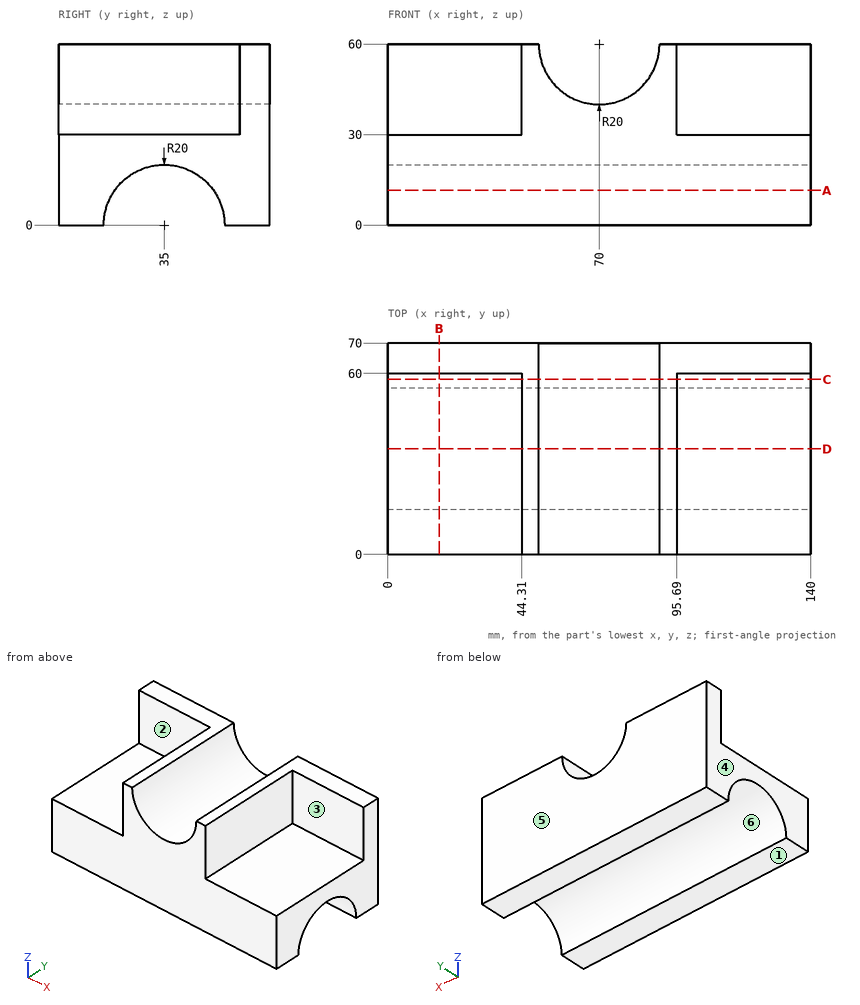
Part print with two shaded views. Sizes in mm from the minimum x, y, z corner. A direction names the side the tool comes from. Coordinates: 2 decimals unless noted, no trailing zeros. Order: outer loops, then holes, each group sorted by start corner. A loop starts at its lowest first (then second) coordinate and runs counter-clockwise, first axis right, second up. Notation, with made-up numbers: (-13, 69) - (9, 69) arc R19 ccw to (9, 90) - close; hole circle Ø4 at (-4, 27.5). An arc over 180 degrees is marked (long way). Write item = value, one per line. Start each with the question number.
1) Two-plate mould, pull along Y, no slides. Class the marked faces 4, 5 and 6: pulls with the +Y half, pulls with the -Y half, needs draft (parallel to the pull), parting line crosses it, or undercut.
2) Saw through at D-D on y = 35. Write the cut outline in (x, z).
3) Saw through at B-B on x = 17. Write the cut outline in (y, z), then the cut area to 3 significant figures.
4) Flat gauge pins, fed straight in: pin 1 Ø1 at (x, z) = (77.5, 9.5) entering from -Y; pin 2 Ø3 at (x, z) = (28.5, 50.5) entering from -Y; pin 3 Ø13.5 at (x, y) = (19.5, 22.5) entering from +Z; pin 4 Ø8 at (y, z) = (43.5, 37) entering from +X. Where does each tip first touch, or does it go through?
5) Saw through at A-A on z = 11.5. Write the cut outline in (x, y), then the cut area to 3 significant figures.
6) 3-axis set-ups, long thin cutter, end or side, ignore diameter. For the marked faces 1, 2 and 3: which of +Z, -Z, +X, -X, +Y, -Y reach the whole face in a straight line?
7) Wall check: line 1 along Y through (x, z) = (79, 4); line 2 along X through (y, z) = (11.5, 52.5); line 3 along X through (y, z) = (45.5, 43) (1 decimal). Give the ranges that are in metal, low to high. Write a range as from..to.
8) Saw through at C-C on y = 58. Write the cut outline in (x, z), then the cut area to 3 significant figures.
From the geometry:
q1.face_4 = needs draft
q1.face_5 = pulls with the +Y half
q1.face_6 = undercut
q2.outline = (0, 20) - (140, 20) - (140, 30) - (95.69, 30) - (95.69, 60) - (90, 60) arc R20 cw to (50, 60) - (44.31, 60) - (44.31, 30) - (0, 30) - close
q3.outline = (0, 0) - (15, 0) arc R20 cw to (55, 0) - (70, 0) - (70, 60) - (60, 60) - (60, 30) - (0, 30) - close
q3.area = 1,770 mm^2
q4.pin_1 = 0
q4.pin_2 = 60
q4.pin_3 = 30
q4.pin_4 = 95.69
q5.outline = (0, 0) - (140, 0) - (140, 18.64) - (0, 18.64) - close; (0, 51.36) - (140, 51.36) - (140, 70) - (0, 70) - close
q5.area = 5,220 mm^2
q6.face_1 = -Z, +X, -X, +Y, -Y
q6.face_2 = +Z, -X, -Y
q6.face_3 = +Z, +X, -Y
q7.line_1 = 0..15.4, 54.6..70
q7.line_2 = 44.31..51.46, 88.54..95.69
q7.line_3 = 44.3..59.5, 80.5..95.7
q8.outline = (0, 0) - (140, 0) - (140, 30) - (95.69, 30) - (95.69, 60) - (90, 60) arc R20 cw to (50, 60) - (44.31, 60) - (44.31, 30) - (0, 30) - close
q8.area = 5,110 mm^2
